from build123d import *

# Parameters (mm, degrees)
BOSS_EXTRUDE1_DEPTH = 5
SKETCH8_R           = 3.5
BOSS_EXTRUDE5_DEPTH = 1.5
SKETCH10_R          = 8
BOSS_EXTRUDE7_DEPTH = 5.75
SKETCH15_R          = 2.8
CUT_EXTRUDE7_DEPTH  = 10
NUT_CUT_START       = -1.5
SKETCH6_W           = 8.4
SKETCH6_H           = 8.4
NUT_CUT_DEPTH       = 46.182751545
SKETCH16_W          = 12
SKETCH16_H          = 3
CUT_EXTRUDE8_DEPTH  = 23
SKETCH17_R          = 2.35
CUT_EXTRUDE9_DEPTH  = 28
CUT_EXTRUDE10_START = 1.5
SKETCH19_R          = 6.25
CUT_EXTRUDE10_DEPTH = 46.182751545
CUT_EXTRUDE11_START = -8
CUT_EXTRUDE11_DEPTH = 3.8
LPATTERN1_COUNT     = 2
LPATTERN1_PITCH     = 10


with BuildPart() as part:
    # Sketch1 → Boss-Extrude1 (new body)
    with BuildSketch(Plane.XY):
        with BuildLine():
            Line((-40.155138696, -0.836255417), (-17.155138696, -0.836255417))
            Line((-17.155138696, -0.836255417), (-5.547811002, -9.922989015))
            ThreePointArc((-5.547811002, -9.922989015), (7.086733598, -8.384066419), (5.547811002, 4.250478181))
            Line((5.547811002, 4.250478181), (-10.947501986, 17.163744583))
            Line((-10.947501986, 17.163744583), (-40.155138696, 17.163744583))
            Line((-40.155138696, 17.163744583), (-40.155138696, -0.836255417))
        make_face()
    extrude(amount=BOSS_EXTRUDE1_DEPTH)

    # Sketch8 → Boss-Extrude5 (add)
    with BuildSketch(Plane.XY.offset(5)):
        with Locations((0, -3.216528208)):
            Circle(SKETCH8_R)
    extrude(amount=BOSS_EXTRUDE5_DEPTH)

    # Sketch10 → section 0 of loft4
    with BuildSketch(Plane.XY.offset(5), mode=Mode.PRIVATE) as loft4_s0:
        with Locations((0, -3.216528208)):
            Circle(SKETCH10_R)
    # loft up to a face of the part (loft4)
    loft([loft4_s0.sketch, part.faces().sort_by_distance((0, -3.216528208, 6.5))[0]])

    # Sketch14 → Boss-Extrude7 (add)
    with BuildSketch(Plane.XY.offset(5)):
        with BuildLine():
            Line((-40.155138696, -0.836255417), (-40.155138696, 17.163744583))
            Line((-40.155138696, 17.163744583), (-10.947501986, 17.163744583))
            Line((-10.947501986, 17.163744583), (0.567762259, 8.149082357))
            ThreePointArc((0.567762259, 8.149082357), (-8.661563286, 3.944402474), (-10.527859744, -6.024384839))
            Line((-10.527859744, -6.024384839), (-17.155138696, -0.836255417))
            Line((-17.155138696, -0.836255417), (-40.155138696, -0.836255417))
        make_face()
    extrude(amount=BOSS_EXTRUDE7_DEPTH)

    # Sketch15 → Cut-Extrude7 (cut)
    with BuildSketch(Plane(origin=(0, 0, 0), x_dir=(-1, 0, 0), z_dir=(0, 0, -1))):
        with Locations((0, -2.836255417)):
            Circle(SKETCH15_R)
    extrude(amount=-CUT_EXTRUDE7_DEPTH, mode=Mode.SUBTRACT)

    # Mirror1: part across plane


with BuildPart() as part_1:
    add(part.part)
    add(part.part.mirror(Plane(origin=(0, -2.836255417, 10.75), x_dir=(1, 0, 0), z_dir=(0, 0, 1))))

    # Sketch6 → nut-cut (cut, through all)
    with BuildSketch(Plane.XY.offset(5).offset(NUT_CUT_START)):
        with Locations((0, -2.836255417)):
            Rectangle(SKETCH6_W, SKETCH6_H)
    extrude(amount=-NUT_CUT_DEPTH, mode=Mode.SUBTRACT)

    # Sketch16 → Cut-Extrude8 (cut)
    with BuildSketch(Plane.ZY.offset(40.155138696)):
        with Locations((10.75, 0.663744583)):
            Rectangle(SKETCH16_W, SKETCH16_H)
        with Locations((10.75, 15.663744583)):
            Rectangle(SKETCH16_W, SKETCH16_H)
    extrude(amount=-CUT_EXTRUDE8_DEPTH, mode=Mode.SUBTRACT)

    # Sketch17 → Cut-Extrude9 (cut)
    with BuildSketch(Plane.ZY.offset(40.155138696)):
        with Locations((10.75, 8.163744583)):
            Circle(SKETCH17_R)
    extrude(amount=-CUT_EXTRUDE9_DEPTH, mode=Mode.SUBTRACT)

    # Sketch19 → Cut-Extrude10 (cut, through all)
    with BuildSketch(Plane.XY.offset(16.5).offset(CUT_EXTRUDE10_START)):
        with Locations(Location((0, -2.836255417, 0), (0, 0, 180))):
            Circle(SKETCH19_R)
    extrude(amount=CUT_EXTRUDE10_DEPTH, mode=Mode.SUBTRACT)

    # Sketch20 → Cut-Extrude11 (cut)
    with BuildSketch(Plane.ZY.offset(40.155138696).offset(CUT_EXTRUDE11_START)):
        Polygon((7, 14.163744583), (14.5, 14.163744583), (14.5, 5.998681073), (10.75, 3.833617564), (7, 5.998681073), align=None)
    cut_extrude11 = extrude(amount=-CUT_EXTRUDE11_DEPTH, mode=Mode.SUBTRACT)

    # LPattern1: Cut-Extrude11 ×2
    with Locations(*[(i * LPATTERN1_PITCH, 0, 0) for i in range(1, LPATTERN1_COUNT)]):
        add(cut_extrude11, mode=Mode.SUBTRACT)


solid = part_1.part
Work out the finished part from the listing and answer in its coordinate system (mm). A direction names the side the tool comes from. Give positions to 0.01 mm unless a question says otherwise; leave off trailing zeros. Write each loop counter-clockwise with the first axis right and the second up, starting at its lowest first coordinate (ties: lowest second). Pieces come first, ordered by that corner, then holes.
Q1. Straight lines are drawn through the part: L1, parallel to X at y = 9.25, z = 7.5; L2, parallel to Z at x = -32.5, y = 8.25; L3, parallel to Y at x = -36.5, z = 10.75. For each, find the intervals that lie inside material, in ascending order.
Answer:
L1: x = -40.16 to -32.16, -28.36 to -22.16, -18.36 to -0.84
L2: z = 0 to 8.4, 13.1 to 21.5
L3: y = 2.16 to 5.81, 10.51 to 14.16
Q2. For a pull along Z with two mould halves and no side action, classify faces 6 (the face through (-1, 0, 18)), 7 (the face through (-20, 10, 14.5)), 8 (the face through (-3, -3, 3.5)) as released by +Z, released by -Z, zero draft, split by the parting line, or undercut.
Answer:
face 6: released by +Z
face 7: undercut
face 8: released by -Z
Q3. The part is cut by section B-B on x = -36. Give the vertices of the cut face in (y, z).
Answer:
outline: (-0.84, 0) - (17.16, 0) - (17.16, 4.75) - (14.16, 4.75) - (14.16, 16.75) - (17.16, 16.75) - (17.16, 21.5) - (-0.84, 21.5) - (-0.84, 16.75) - (2.16, 16.75) - (2.16, 4.75) - (-0.84, 4.75) - close; hole circle Ø4.7 at (8.16, 10.75)
Q4. The part is cut by section C-C on x = 0. State how many separate pieces and enclosed holes the cut face has, and give its area (3 significant figures).
Answer:
separate pieces: 3
enclosed holes: 0
area: 137 mm2
Q5. Given pin 1 (4 mm diameter, centred on y = -5.5, z = 7, fed in from -X); pin 2 (2 mm diameter, centred on y = 11, z = 9, fed in from +X); pin 3 (7.5 mm diameter, centred on x = 0, y = -2.84, fed in from +Z), each flat-ended and moving along its own axis, determine where each tip first touches the part or whether it passes through.
Answer:
pin 1: stops at x = -13.75
pin 2: stops at x = -1.8
pin 3: stops at z = 18
Q6. A tool of negligible diameter and unlimited length cuts with its end or side. For faces 1 (the face through (-36.21, 6.73, 8.89)), 2 (the face through (-29, 2.164, 11)), 3 (the face through (-20.28, 4.93, 12.65)), 4 (the face through (-4.2, -3, 2)), 5 (the face through (-29, 16, 16.75)), from which of +Z, -Z, +X, -X, +Y, -Y can it reach the whole face along a straight path? Write none if from no direction.
Answer:
face 1: -X
face 2: -X, -Y
face 3: +Y
face 4: -Z
face 5: -X, +Y
Q7. The part is cut by section A-A on z = 15.75. Give the vertices of the cut face in (x, y).
Answer:
outline: (-40.16, 2.16) - (-17.16, 2.16) - (-17.16, -0.84) - (-10.53, -6.02) arc R11 cw to (0.57, 8.15) - (-10.95, 17.16) - (-17.16, 17.16) - (-17.16, 14.16) - (-40.16, 14.16) - close; circle Ø11.5 at (0, -3.22); hole circle Ø5.6 at (0, -2.84)
